from build123d import *

# Parameters (mm, degrees)
F0_W     = 152.3896604776
F0_H     = 152.2873565555
F1_DEPTH = 25.4
F3_DEPTH = 50.8
F5_DEPTH = 25.4
F7_DEPTH = 50.8
F8_DEPTH = 25.4
F9_DEPTH = 68.072


with BuildPart() as f1:
    # F0 (on Top) → F1 (new body)
    with BuildSketch(Plane.XY):
        with Locations((0.0336691737, 0.0013746321)):
            Rectangle(F0_W, F0_H)
    extrude(amount=F1_DEPTH)

    # F2 (on face) → F3 (join)
    with BuildSketch(Plane.XY.offset(25.4)):
        Polygon((-49.0896850824, 12.7), (-49.0896850824, 0), (-49.0896850824, -12.7), (27.879094705, -12.7), (27.879094705, 12.7), align=None)
    extrude(amount=F3_DEPTH)

    # F4 (on face) → F5 (cut)
    with BuildSketch(Plane.XZ.offset(12.7)):
        Polygon((-49.0896850824, 25.4), (27.879094705, 76.2), (-49.0896850824, 76.2), align=None)
    extrude(amount=-F5_DEPTH, mode=Mode.SUBTRACT)

    # F6 (on face) → F7 (join)
    with BuildSketch(Plane.XY.offset(25.4)):
        with BuildLine():
            Line((27.879094705, 12.7), (27.879094705, -12.7))
            ThreePointArc((27.879094705, -12.7), (43.9814429182, -50.5730961069), (76.2284994125, -76.1423036456))
            Line((76.2284994125, -76.1423036456), (76.2284994125, -47.5807675257))
            ThreePointArc((76.2284994125, -47.5807675257), (51.7952412993, 0.0013746321), (76.2284994125, 47.5835167899))
            Line((76.2284994125, 47.5835167899), (76.2284994125, 76.1450529099))
            ThreePointArc((76.2284994125, 76.1450529099), (43.9805998825, 50.5747391516), (27.8786713028, 12.7))
            Line((27.8786713028, 12.7), (27.879094705, 12.7))
        make_face()
        with BuildLine():
            Line((76.2284994125, -47.5807675257), (76.2284994125, -76.1423036456))
            ThreePointArc((76.2284994125, -76.1423036456), (155.7044526061, -70.0276226689), (193.7801140773, 0.0013746321))
            ThreePointArc((193.7801140773, 0.0013746321), (155.7044526061, 70.0303719332), (76.2284994125, 76.1450529099))
            Line((76.2284994125, 76.1450529099), (76.2284994125, 47.5835167899))
            ThreePointArc((76.2284994125, 47.5835167899), (137.0877616024, 52.084244528), (168.8915508086, 0.0013746321))
            ThreePointArc((168.8915508086, 0.0013746321), (137.0877616024, -52.0814952637), (76.2284994125, -47.5807675257))
        make_face()
    extrude(amount=F7_DEPTH)

    # F8 (add): a face of the model
    f8_faces = [f1.faces().sort_by_distance(p)[0] for p in [
        (191.7389103695, 0.0013746321, 25.4),
    ]]
    extrude(f8_faces, amount=F8_DEPTH)

    # F9 (cut): a face of the model
    f9_faces = [f1.faces().sort_by_distance(p)[0] for p in [
        (66.2561526249, 0.0013746321, 25.4),
    ]]
    extrude(f9_faces, amount=-F9_DEPTH, mode=Mode.SUBTRACT)


solid = f1.part
For this review, take the finished solid that the model builds, in its own axes (mm). A direction names the side the tool comes from. Give positions to 0.01 mm unless a question says otherwise; leave off trailing zeros. Loops run counter-clockwise (first coordinate to the right, second up) from the corner with the lowest first, then second, coordinate; pieces in that order, holes last.
Item 1: Take a section at C-C, the plane x = 145. State the section outline as (y, z) points.
Item 2: Take a section at A-A, the plane z = 12. State the section outline as (x, y) points, and give its area (3 significant figures).
Item 3: For line 1 along Y through (x, z) = (109, 68.5); line 2 along X through (y, z) = (-27, 32); line 3 along X through (y, z) = (41, 54), list the stretches that pass through material, from the lowest coordinate up.
Item 4: Take a section at D-D, the plane y = 24.5. State the section outline as (x, z) points.
Item 5: Insertion check: pin 1 (4 mm diameter, centred on y = -44, z = 24, fed in from +X); pin 2 (12 mm diameter, centred on x = -24, y = -43, fed in from +Z); pin 3 (12.5 mm diameter, centred on x = 17, z = 11, fed in from +Y). Each pin has a flat end and moves straight along its axis. Give the tip position at first contact, or say it passes through.
Item 6: Take a section at B-B, the plane y = -4.5. State the section outline as (x, z) points, and give its area (3 significant figures).
Item 7: Tool access review of faces 1 (the flat face through (6, -12.7, 39)), 2 (the flat face through (-2, 12.7, 45)), 3 (the flat face through (-1, -76.142, 13)), 4 (the flat face through (-18, 18, 25.4)), 5 (the flat face through (-1, 76.145, 13)): name each direction out of +Z, -Z, +X, -X, +Y, -Y from which nothing blocks a thin tool from reaching the whole face with its end or side.
Calculated:
1. outline: (-75.9, 0) - (-47.19, 0) - (-47.19, 76.2) - (-75.9, 76.2) - close; (47.19, 0) - (75.9, 0) - (75.9, 76.2) - (47.19, 76.2) - close
2. outline: (-76.16, -76.14) - (76.23, -76.14) arc R83.44 ccw (long way) to (76.23, 76.15) - (-76.16, 76.15) - close; hole circle Ø117.1 at (110.34, 0)
2. area: 28,900 mm2
3. line 1: y = -83.42 to -58.53, 58.53 to 83.43
3. line 2: x = 31.4 to 58.39, 162.29 to 189.29
3. line 3: x = 37.67 to 68.55, 152.14 to 183.01
4. outline: (-76.16, 0) - (57.17, 0) - (57.17, 76.2) - (30.58, 76.2) - (30.58, 25.4) - (-76.16, 25.4) - close; (163.52, 0) - (190.1, 0) - (190.1, 76.2) - (163.52, 76.2) - close
5. pin 1: stops at x = 182.44
5. pin 2: stops at z = 25.4
5. pin 3: stops at y = 76.15
6. outline: (-76.16, 0) - (51.97, 0) - (51.97, 76.2) - (27.88, 76.2) - (-49.09, 25.4) - (-76.16, 25.4) - close; (168.72, 0) - (193.66, 0) - (193.66, 76.2) - (168.72, 76.2) - close
6. area: 8,330 mm2
7. face 1: +Z, -X, -Y
7. face 2: +Z, -X, +Y
7. face 3: +Z, -Z, -X, -Y
7. face 4: +Z, -X
7. face 5: +Z, -Z, -X, +Y
